Design review of the part built by this model. Coordinates are the model's own, in mm. A direction names the side the tool comes from. Coordinates: 2 decimals unless noted, no trailing zeros. Loops run counter-clockwise (first coordinate to the right, second up) from the corner with the lowest first, then second, coordinate; pieces in that order, holes last. Notation, with made-up numbers: (26, 41) -> (48, 41) arc R14 ccw to (48, 59) -> close; hole circle Ø10 at (-14.75, 21.5). An arc over 180 degrees is marked (long way). Answer in a Markdown table with one row per item.
```python
from build123d import *

# Parameters (mm, degrees)
CONVERT_SOLID1_START       = -5
CONVERT_SOLID1_OUTLINE_R   = 1.65
CONVERT_SOLID1_OUTLINE_R_2 = 10.75
CONVERT_SOLID1_OUTLINE_R_3 = 1.25
CONVERT_SOLID1_OUTLINE_R_4 = 1.5
CONVERT_SOLID1_OUTLINE_R_5 = 5
CONVERT_SOLID1_OUTLINE_R_6 = 12
CONVERT_SOLID1_DEPTH       = 5


# Read off the part's stored shape, not the designer's step: Convert-Solid1
with BuildPart() as part:
    # Convert-Solid1 outline → Convert-Solid1 (new body)
    with BuildSketch(Plane.XY.offset(CONVERT_SOLID1_START)):
        with BuildLine():
            ThreePointArc((19.5, 254.5), (5.711417767, 248.788582233), (0, 235))
            Line((0, 235), (0, 3))
            ThreePointArc((0, 3), (0.878679656, 0.878679656), (3, 0))
            Line((3, 0), (238, 0))
            ThreePointArc((238, 0), (240.121320344, 0.878679656), (241, 3))
            Line((241, 3), (241, 235))
            ThreePointArc((241, 235), (235.288582233, 248.788582233), (221.5, 254.5))
            Line((221.5, 254.5), (19.5, 254.5))
        make_face()
        with Locations((6.25, 6.25)):
            Circle(CONVERT_SOLID1_OUTLINE_R, mode=Mode.SUBTRACT)
        with Locations((16.75, 10.75)):
            Circle(CONVERT_SOLID1_OUTLINE_R, mode=Mode.SUBTRACT)
        with Locations((28, 22)):
            Circle(CONVERT_SOLID1_OUTLINE_R_2, mode=Mode.SUBTRACT)
        with Locations((39.25, 10.75)):
            Circle(CONVERT_SOLID1_OUTLINE_R, mode=Mode.SUBTRACT)
        with Locations((49.75, 6.25)):
            Circle(CONVERT_SOLID1_OUTLINE_R, mode=Mode.SUBTRACT)
        with Locations((6.25, 37.75)):
            Circle(CONVERT_SOLID1_OUTLINE_R, mode=Mode.SUBTRACT)
        with Locations((16.75, 33.25)):
            Circle(CONVERT_SOLID1_OUTLINE_R, mode=Mode.SUBTRACT)
        with Locations((18.75, 53)):
            Circle(CONVERT_SOLID1_OUTLINE_R, mode=Mode.SUBTRACT)
        with Locations((39.25, 33.25)):
            Circle(CONVERT_SOLID1_OUTLINE_R, mode=Mode.SUBTRACT)
        with Locations((49.75, 37.75)):
            Circle(CONVERT_SOLID1_OUTLINE_R, mode=Mode.SUBTRACT)
        with Locations((89.75, 6.25)):
            Circle(CONVERT_SOLID1_OUTLINE_R, mode=Mode.SUBTRACT)
        with Locations((69.75, 22)):
            Circle(CONVERT_SOLID1_OUTLINE_R, mode=Mode.SUBTRACT)
        with Locations((82.5, 22)):
            Circle(CONVERT_SOLID1_OUTLINE_R_3, mode=Mode.SUBTRACT)
        with Locations((105, 7.5)):
            Circle(CONVERT_SOLID1_OUTLINE_R_4, mode=Mode.SUBTRACT)
        with Locations((89.75, 37.75)):
            Circle(CONVERT_SOLID1_OUTLINE_R, mode=Mode.SUBTRACT)
        with Locations((105, 38.5)):
            Circle(CONVERT_SOLID1_OUTLINE_R_4, mode=Mode.SUBTRACT)
        with Locations((6.25, 68.25)):
            Circle(CONVERT_SOLID1_OUTLINE_R, mode=Mode.SUBTRACT)
        with Locations((19.5, 83)):
            Circle(CONVERT_SOLID1_OUTLINE_R_5, mode=Mode.SUBTRACT)
        with Locations((31.75, 83)):
            Circle(CONVERT_SOLID1_OUTLINE_R, mode=Mode.SUBTRACT)
        with Locations((6.25, 97.75)):
            Circle(CONVERT_SOLID1_OUTLINE_R, mode=Mode.SUBTRACT)
        with Locations((18.75, 117.75)):
            Circle(CONVERT_SOLID1_OUTLINE_R, mode=Mode.SUBTRACT)
        with Locations((136, 7.5)):
            Circle(CONVERT_SOLID1_OUTLINE_R_4, mode=Mode.SUBTRACT)
        with Locations((120.5, 23)):
            Circle(CONVERT_SOLID1_OUTLINE_R_6, mode=Mode.SUBTRACT)
        with Locations((151.25, 6.25)):
            Circle(CONVERT_SOLID1_OUTLINE_R, mode=Mode.SUBTRACT)
        with Locations((171.25, 22)):
            Circle(CONVERT_SOLID1_OUTLINE_R, mode=Mode.SUBTRACT)
        with Locations((136, 38.5)):
            Circle(CONVERT_SOLID1_OUTLINE_R_4, mode=Mode.SUBTRACT)
        with Locations((151.25, 37.75)):
            Circle(CONVERT_SOLID1_OUTLINE_R, mode=Mode.SUBTRACT)
        with Locations((191.25, 6.25)):
            Circle(CONVERT_SOLID1_OUTLINE_R, mode=Mode.SUBTRACT)
        with Locations((201.75, 10.75)):
            Circle(CONVERT_SOLID1_OUTLINE_R, mode=Mode.SUBTRACT)
        with Locations((224.25, 10.75)):
            Circle(CONVERT_SOLID1_OUTLINE_R, mode=Mode.SUBTRACT)
        with Locations((234.75, 6.25)):
            Circle(CONVERT_SOLID1_OUTLINE_R, mode=Mode.SUBTRACT)
        with Locations((213, 22)):
            Circle(CONVERT_SOLID1_OUTLINE_R_2, mode=Mode.SUBTRACT)
        with Locations((191.25, 37.75)):
            Circle(CONVERT_SOLID1_OUTLINE_R, mode=Mode.SUBTRACT)
        with Locations((201.75, 33.25)):
            Circle(CONVERT_SOLID1_OUTLINE_R, mode=Mode.SUBTRACT)
        with Locations((224.25, 33.25)):
            Circle(CONVERT_SOLID1_OUTLINE_R, mode=Mode.SUBTRACT)
        with Locations((234.75, 37.75)):
            Circle(CONVERT_SOLID1_OUTLINE_R, mode=Mode.SUBTRACT)
        with Locations((222.25, 53)):
            Circle(CONVERT_SOLID1_OUTLINE_R, mode=Mode.SUBTRACT)
        with Locations((209.25, 83)):
            Circle(CONVERT_SOLID1_OUTLINE_R, mode=Mode.SUBTRACT)
        with Locations((234.75, 68.25)):
            Circle(CONVERT_SOLID1_OUTLINE_R, mode=Mode.SUBTRACT)
        with Locations((221.5, 83)):
            Circle(CONVERT_SOLID1_OUTLINE_R_5, mode=Mode.SUBTRACT)
        with Locations((234.75, 97.75)):
            Circle(CONVERT_SOLID1_OUTLINE_R, mode=Mode.SUBTRACT)
        with Locations((222.25, 117.75)):
            Circle(CONVERT_SOLID1_OUTLINE_R, mode=Mode.SUBTRACT)
        with Locations((6.25, 137.75)):
            Circle(CONVERT_SOLID1_OUTLINE_R, mode=Mode.SUBTRACT)
        with Locations((18.75, 157.75)):
            Circle(CONVERT_SOLID1_OUTLINE_R, mode=Mode.SUBTRACT)
        with Locations((6.25, 177.75)):
            Circle(CONVERT_SOLID1_OUTLINE_R, mode=Mode.SUBTRACT)
        with Locations((18.75, 197.75)):
            Circle(CONVERT_SOLID1_OUTLINE_R, mode=Mode.SUBTRACT)
        with Locations((6.25, 216.291713066)):
            Circle(CONVERT_SOLID1_OUTLINE_R, mode=Mode.SUBTRACT)
        with Locations((7.25, 235)):
            Circle(CONVERT_SOLID1_OUTLINE_R, mode=Mode.SUBTRACT)
        with Locations((28.16205807, 226.33794193)):
            Circle(CONVERT_SOLID1_OUTLINE_R, mode=Mode.SUBTRACT)
        with Locations((19.5, 235)):
            Circle(CONVERT_SOLID1_OUTLINE_R_5, mode=Mode.SUBTRACT)
        with Locations((19.5, 247.25)):
            Circle(CONVERT_SOLID1_OUTLINE_R, mode=Mode.SUBTRACT)
        with Locations((38.208286934, 248.25)):
            Circle(CONVERT_SOLID1_OUTLINE_R, mode=Mode.SUBTRACT)
        with Locations((60.5, 235.75)):
            Circle(CONVERT_SOLID1_OUTLINE_R, mode=Mode.SUBTRACT)
        with Locations((80.5, 248.25)):
            Circle(CONVERT_SOLID1_OUTLINE_R, mode=Mode.SUBTRACT)
        with Locations((100.5, 235.75)):
            Circle(CONVERT_SOLID1_OUTLINE_R, mode=Mode.SUBTRACT)
        with BuildLine():
            Line((201, 46), (40, 46))
            ThreePointArc((40, 46), (29.393398282, 50.393398282), (25, 61))
            Line((25, 61), (25, 62.167333344))
            ThreePointArc((25, 62.167333344), (25.51002008, 63.840653397), (26.866666667, 64.945022231))
            ThreePointArc((26.866666667, 64.945022231), (39, 83), (26.866666667, 101.054977769))
            ThreePointArc((26.866666667, 101.054977769), (25.51002008, 102.159346603), (25, 103.832666656))
            Line((25, 103.832666656), (25, 214.167333344))
            ThreePointArc((25, 214.167333344), (25.51002008, 215.840653397), (26.866666667, 216.945022231))
            ThreePointArc((26.866666667, 216.945022231), (33.288582233, 221.211417767), (37.554977769, 227.633333333))
            ThreePointArc((37.554977769, 227.633333333), (38.659346603, 228.98997992), (40.332666656, 229.5))
            Line((40.332666656, 229.5), (200.667333344, 229.5))
            ThreePointArc((200.667333344, 229.5), (202.340653397, 228.98997992), (203.445022231, 227.633333333))
            ThreePointArc((203.445022231, 227.633333333), (207.711417767, 221.211417767), (214.133333333, 216.945022231))
            ThreePointArc((214.133333333, 216.945022231), (215.48997992, 215.840653397), (216, 214.167333344))
            Line((216, 214.167333344), (216, 103.832666656))
            ThreePointArc((216, 103.832666656), (215.48997992, 102.159346603), (214.133333333, 101.054977769))
            ThreePointArc((214.133333333, 101.054977769), (202, 83), (214.133333333, 64.945022231))
            ThreePointArc((214.133333333, 64.945022231), (215.48997992, 63.840653397), (216, 62.167333344))
            Line((216, 62.167333344), (216, 61))
            ThreePointArc((216, 61), (211.606601718, 50.393398282), (201, 46))
        make_face(mode=Mode.SUBTRACT)
        with Locations((234.75, 137.75)):
            Circle(CONVERT_SOLID1_OUTLINE_R, mode=Mode.SUBTRACT)
        with Locations((222.25, 157.75)):
            Circle(CONVERT_SOLID1_OUTLINE_R, mode=Mode.SUBTRACT)
        with Locations((234.75, 177.75)):
            Circle(CONVERT_SOLID1_OUTLINE_R, mode=Mode.SUBTRACT)
        with Locations((140.5, 235.75)):
            Circle(CONVERT_SOLID1_OUTLINE_R, mode=Mode.SUBTRACT)
        with Locations((120.5, 248.25)):
            Circle(CONVERT_SOLID1_OUTLINE_R, mode=Mode.SUBTRACT)
        with Locations((180.5, 235.75)):
            Circle(CONVERT_SOLID1_OUTLINE_R, mode=Mode.SUBTRACT)
        with Locations((160.5, 248.25)):
            Circle(CONVERT_SOLID1_OUTLINE_R, mode=Mode.SUBTRACT)
        with Locations((222.25, 197.75)):
            Circle(CONVERT_SOLID1_OUTLINE_R, mode=Mode.SUBTRACT)
        with Locations((234.75, 216.291713066)):
            Circle(CONVERT_SOLID1_OUTLINE_R, mode=Mode.SUBTRACT)
        with Locations((202.791713066, 248.25)):
            Circle(CONVERT_SOLID1_OUTLINE_R, mode=Mode.SUBTRACT)
        with Locations((212.83794193, 226.33794193)):
            Circle(CONVERT_SOLID1_OUTLINE_R, mode=Mode.SUBTRACT)
        with Locations((221.5, 235)):
            Circle(CONVERT_SOLID1_OUTLINE_R_5, mode=Mode.SUBTRACT)
        with Locations((233.75, 235)):
            Circle(CONVERT_SOLID1_OUTLINE_R, mode=Mode.SUBTRACT)
        with Locations((221.5, 247.25)):
            Circle(CONVERT_SOLID1_OUTLINE_R, mode=Mode.SUBTRACT)
    extrude(amount=CONVERT_SOLID1_DEPTH)


solid = part.part
```
(1) Tool access review of faces 1 (the flat face through (119, 44, 0)), 2 (the cylindrical face through (33.212, 221.135, -2.535)): name each direction out of +Z, -Z, +X, -X, +Y, -Y from which nothing blocks a thin tool from reaching the whole face with its end or side.
Evaluation:
| item | result |
|---|---|
| face 1 | +Z, +X, -X, +Y, -Y |
| face 2 | +Z, -Z |
(2) Take a section at C-C on z = -4.2. Count the separate pieces of the cut face and the enclosed holes in it, and give its area (3 significant figures).
Evaluation:
| item | result |
|---|---|
| separate pieces | 1 |
| enclosed holes | 70 |
| area | 25,200 mm² |
(3) Draft analysis for pull direction Y (two halves, no side actions). For faces 3 (the cylindrical face through (235.439, 248.636, -2.535)), 4 (the cylindrical face through (108.51, 23.53, -2.54)), 5 (the flat face through (119, 44, -5)), state which applies: pulls with the +Y half, pulls with the -Y half, needs draft (parallel to the pull), parting line crosses it, or undercut.
Evaluation:
| item | result |
|---|---|
| face 3 | pulls with the +Y half |
| face 4 | undercut |
| face 5 | needs draft |
(4) Take a section at A-A on y = 28.5. Give the boundary of the cut face in (x, z).
Evaluation:
| item | result |
|---|---|
| outline | (0, -5) -> (19.44, -5) -> (19.44, 0) -> (0, 0) -> close; (36.56, -5) -> (109.83, -5) -> (109.83, 0) -> (36.56, 0) -> close; (131.17, -5) -> (204.44, -5) -> (204.44, 0) -> (131.17, 0) -> close; (221.56, -5) -> (241, -5) -> (241, 0) -> (221.56, 0) -> close |
(5) For pin 1 (4 mm diameter, centred on x = 39.25, y = 10.75, fed in from -Z), flat-tipped, find the tip position at first contact; note if it passes through.
Evaluation:
| item | result |
|---|---|
| pin 1 | stops at z = -5 |
(6) To check wall thickness, follow probe 1 along Y at (x, z) = (191, -4.15); probe 2 along Y at (x, z) = (120.5, -2.35); probe 3 along Y at (x, z) = (82.5, -1.1). State the ranges of each line that lie inside material, in increasing order.
Evaluation:
| item | result |
|---|---|
| probe 1 | y = 0 to 4.62, 7.88 to 36.12, 39.38 to 46, 229.5 to 254.5 |
| probe 2 | y = 0 to 11, 35 to 46, 229.5 to 246.6, 249.9 to 254.5 |
| probe 3 | y = 0 to 20.75, 23.25 to 46, 229.5 to 254.5 |
(7) Take a section at B-B on y = 148. Give the boundary of the cut face in (x, z).
Evaluation:
| item | result |
|---|---|
| outline | (0, -5) -> (25, -5) -> (25, 0) -> (0, 0) -> close; (216, -5) -> (241, -5) -> (241, 0) -> (216, 0) -> close |
